from build123d import *

# Parameters (mm, degrees)
SKETCH1_W           = 150
SKETCH1_H           = 80
BOSS_EXTRUDE4_DEPTH = 50
SKETCH2_W           = 145
SKETCH2_H           = 75
CUT_EXTRUDE12_DEPTH = 45
SKETCH3_R           = 2.5
CUT_EXTRUDE13_DEPTH = 99.615414617


with BuildPart() as part:
    # Sketch1 → Boss-Extrude4 (new body)
    with BuildSketch(Plane(origin=(0, 0, 0), x_dir=(1, 0, 0), z_dir=(0, 1, 0))):
        Rectangle(SKETCH1_W, SKETCH1_H)
    extrude(amount=BOSS_EXTRUDE4_DEPTH)

    # Sketch2 → Cut-Extrude12 (cut)
    with BuildSketch(Plane(origin=(0, 0, 0), x_dir=(1, 0, 0), z_dir=(0, 1, 0))):
        Rectangle(SKETCH2_W, SKETCH2_H)
    extrude(amount=CUT_EXTRUDE12_DEPTH, mode=Mode.SUBTRACT)

    # Sketch3 → Cut-Extrude13 (cut, through all)
    with BuildSketch(Plane(origin=(0, 0, 0), x_dir=(1, 0, 0), z_dir=(0, 1, 0))):
        with Locations(Location((0, 0, 0), (0, 0, 270))):
            Circle(SKETCH3_R)
    extrude(amount=CUT_EXTRUDE13_DEPTH, mode=Mode.SUBTRACT)


solid = part.part
The listing builds one solid part. Answer for the finished solid, in the listing's coordinates (mm). A direction names the side the tool comes from. Round coordinates to 2 decimals unless told otherwise and drop trailing zeros. Order: outer loops, then holes, each group sorted by start corner. A loop starts at its lowest first (then second) coordinate and runs counter-clockwise, first axis right, second up. Notation, with made-up numbers: (1, -27) -> (15, -27) arc R19 ccw to (15, 2) -> close; hole circle Ø9 at (-4.5, 69). An arc over 180 degrees is marked (long way). One line per item, written item: value.
Item 1: For faces 4 (the flat face through (-1, 50, -9)), 5 (the flat face through (-72.5, 22, 1)), determine the directions among +Z, -Z, +X, -X, +Y, -Y from which every point of the face is accessible in a straight line to the end or side of a thin tool.
Taken from the geometry:
face 4: +Z, -Z, +X, -X, +Y
face 5: -Y
Item 2: Find section C-C, the plane x = 0. Give the vertices of the cut face in (y, z).
Taken from the geometry:
outline: (0, -40) -> (50, -40) -> (50, -2.5) -> (45, -2.5) -> (45, -37.5) -> (0, -37.5) -> close; (0, 37.5) -> (45, 37.5) -> (45, 2.5) -> (50, 2.5) -> (50, 40) -> (0, 40) -> close
Item 3: Given P1, Ø5, axis at x = 9, z = -23.5, coming from the -Y side; P2, Ø3, axis at x = 0, z = 0, coming from the +Y side, each flat-ended and moving along its own axis, determine where each tip first touches the part or whether it passes through.
Taken from the geometry:
P1: stops at y = 45
P2: passes through
Item 4: Straight lines are drawn through the part: L1, parallel to X at y = 15, z = -0.5; L2, parallel to Z at x = 8.5, y = 17; L3, parallel to X at y = 48.65, z = 0. For each, find the intervals that lie inside material, in ascending order.
Taken from the geometry:
L1: x = -75 to -72.5, 72.5 to 75
L2: z = -40 to -37.5, 37.5 to 40
L3: x = -75 to -2.5, 2.5 to 75
Item 5: Find section D-D, the plane x = -41. Give the vertices of the cut face in (y, z).
Taken from the geometry:
outline: (0, -40) -> (50, -40) -> (50, 40) -> (0, 40) -> (0, 37.5) -> (45, 37.5) -> (45, -37.5) -> (0, -37.5) -> close
Item 6: Find section B-B, the plane y = 26. Give the vertices of the cut face in (x, z), then the cut area to 4 significant figures.
Taken from the geometry:
outline: (-75, -40) -> (75, -40) -> (75, 40) -> (-75, 40) -> close; hole (-72.5, -37.5) -> (72.5, -37.5) -> (72.5, 37.5) -> (-72.5, 37.5) -> close
area: 1,125 mm2
Item 7: Find section A-A, the plane z = 0. Give the vertices of the cut face in (x, y).
Taken from the geometry:
outline: (-75, 0) -> (-72.5, 0) -> (-72.5, 45) -> (-2.5, 45) -> (-2.5, 50) -> (-75, 50) -> close; (2.5, 45) -> (72.5, 45) -> (72.5, 0) -> (75, 0) -> (75, 50) -> (2.5, 50) -> close
Item 8: For a pull along X with two mould halves and no side action, classify faces 1 (the cylindrical face through (-2.44, 47.46, -0.54)), 2 (the flat face through (75, 25, 1)), 3 (the flat face through (-1, 25, -40)) as released by +X, released by -X, zero draft, split by the parting line, or undercut.
Taken from the geometry:
face 1: undercut
face 2: released by +X
face 3: zero draft
